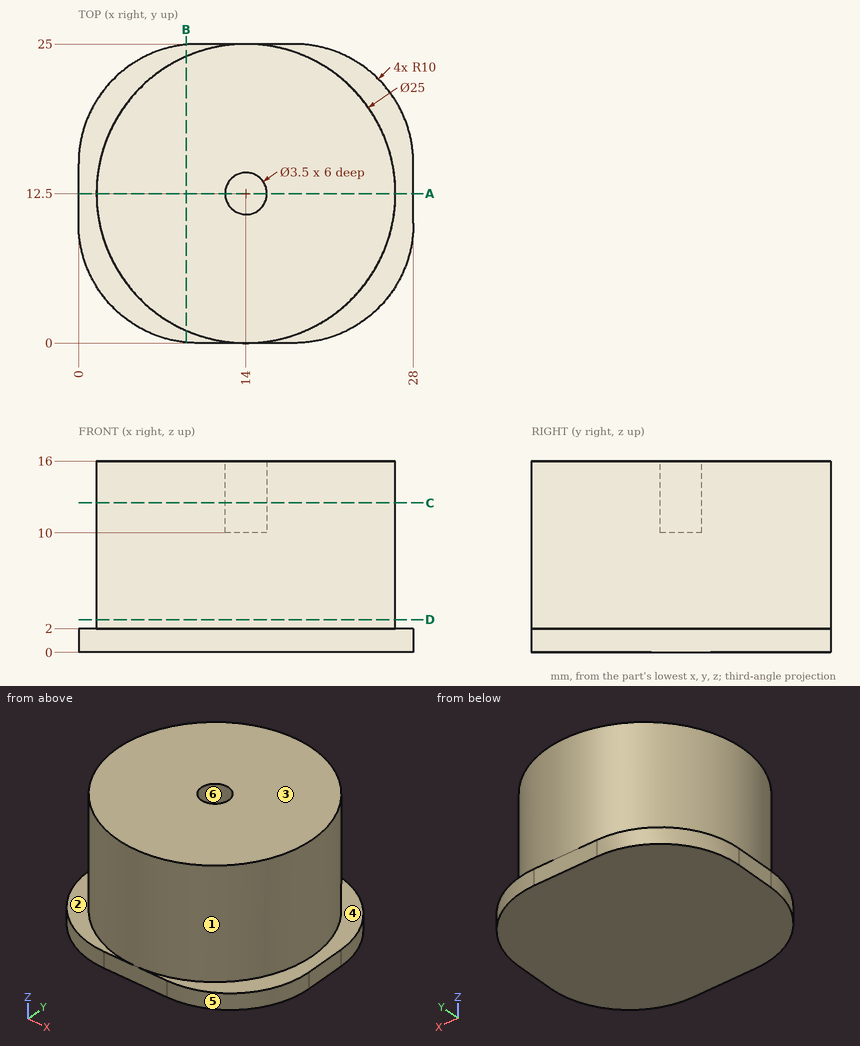
Study the drawing (mm; zero at the part's minimum x, y, z) and answer. A direction names the side the tool comes from. Give positions to 0.01 mm unless a question says otherwise; leave off trailing zeros. Write each loop counter-clockwise with the first axis right and the second up, starting at its lowest first coordinate (ties: lowest second). Pieces come first, ordered by that corner, then holes.
Item 1: Section A-A, the plane y = 12.5 is taken. Write down the section's boundary in (x, z).
Item 2: Section D-D, the plane z = 2.75 is taken. Write down the section's boundary in (x, y).
Item 3: Find the intervals of material crossed by line 1 along Y through (x, z) = (14, 14.6); line 2 along Z through (x, y) = (3.5, 3.5); line 3 along Y through (x, z) = (21.75, 2.75), in increasing order.
Item 4: Determine the mould class of the marked faces 4, 5 and 6 for opening direction X: released by +X, released by -X, zero draft, split by the parting line, or undercut.
Item 5: Section C-C, the plane z = 12.5 is taken. Write down the section's boundary in (x, y), plus the area to 3 significant figures.
Item 6: Which of the six approach directions +Z, -Z, +X, -X, +Y, -Y give full straight-line access (tool end or side, diameter ignored) to the marked faces 1, 2 and 3?
Item 7: Section B-B, the plane x = 9 is taken. Write down the section's boundary in (y, z), plus the area to 3 significant figures.
Item 8: Flat-ended cylindrical pins translate along their axes: P1, Ø8, axis at y = 16, z = 7.5, coming from the +X side; P2, Ø1, axis at y = 5.5, z = 11, coming from the +X side; P3, Ø1, axis at y = 15, z = 7, coming from the +X side. Find the tip coordinate at first contact, or state that the pin passes through.
Completed:
1. outline: (0, 0) - (28, 0) - (28, 2) - (26.5, 2) - (26.5, 16) - (15.75, 16) - (15.75, 10) - (12.25, 10) - (12.25, 16) - (1.5, 16) - (1.5, 2) - (0, 2) - close
2. outline: circle Ø25 at (14, 12.5)
3. line 1: y = 0 to 10.75, 14.25 to 25
3. line 2: z = 0 to 2
3. line 3: y = 2.69 to 22.31
4. face 4: zero draft
4. face 5: released by +X
4. face 6: undercut
5. outline: circle Ø25 at (14, 12.5); hole circle Ø3.5 at (14, 12.5)
5. area: 481 mm2
6. face 1: +Z
6. face 2: +Z, -X
6. face 3: +Z, +X, -X, +Y, -Y
7. outline: (0.05, 0) - (24.95, 0) - (24.95, 2) - (23.96, 2) - (23.96, 16) - (1.04, 16) - (1.04, 2) - (0.05, 2) - close
7. area: 371 mm2
8. P1: stops at x = 26.5
8. P2: stops at x = 24.68
8. P3: stops at x = 26.34
